from build123d import *

# Parameters (mm, degrees)
F0_W           = 51
F0_H           = 56
F0_W_2         = 47
F0_H_2         = 52
F1_DEPTH       = 1.5
F2_R           = 5
F3_DEPTH       = 3
F5_D           = 2
F5_CBORE_D     = 3.7
F5_CBORE_DEPTH = 1
F7_DEPTH       = 1.5


with BuildPart() as f1:
    # F0 (on Front) → F1 (new body)
    with BuildSketch(Plane.XZ):
        with Locations((25.5, 28)):
            Rectangle(F0_W, F0_H)
        with Locations((25.5, 28)):
            Rectangle(F0_W_2, F0_H_2, mode=Mode.SUBTRACT)
        with Locations((25.5, 28)):
            Rectangle(F0_W_2, F0_H_2)
    extrude(amount=F1_DEPTH)

    # F2
    f2_edges = [f1.edges().sort_by_distance(p)[0] for p in [
        (0, -0.75, 56),
        (51, -0.75, 56),
        (51, -0.75, 0),
        (0, -0.75, 0),
    ]]
    fillet(f2_edges, radius=F2_R)

    # F0 (on Front) → F3 (join)
    with BuildSketch(Plane.XZ):
        with Locations((25.5, 28)):
            Rectangle(F0_W_2, F0_H_2)
    extrude(amount=F3_DEPTH)

    # F5 (through all)
    with Locations(Plane(origin=(0, 0, 0), x_dir=(1, 0, 0), z_dir=(0, 1, 0))):
        with Locations((47.75, -52.75), (3.25, -52.75), (47.75, -3.25), (3.25, -3.25)):
            CounterBoreHole(F5_D / 2, F5_CBORE_D / 2, F5_CBORE_DEPTH)

    # F6 (on face) → F7 (cut)
    with BuildSketch(Plane.XZ.offset(3)):
        with BuildLine():
            Line((2, 54), (2, 50.2))
            ThreePointArc((2, 50.2), (4.6870057685, 51.3129942315), (5.8, 54))
            Line((5.8, 54), (2, 54))
        make_face()
        with BuildLine():
            ThreePointArc((45.2, 54), (46.3129942315, 51.3129942315), (49, 50.2))
            Line((49, 50.2), (49, 54))
            Line((49, 54), (45.2, 54))
        make_face()
        with BuildLine():
            Line((49, 2), (49, 5.8))
            ThreePointArc((49, 5.8), (46.3129942315, 4.6870057685), (45.2, 2))
            Line((45.2, 2), (49, 2))
        make_face()
        with BuildLine():
            ThreePointArc((5.8, 2), (4.6870057685, 4.6870057685), (2, 5.8))
            Line((2, 5.8), (2, 2))
            Line((2, 2), (5.8, 2))
        make_face()
    extrude(amount=-F7_DEPTH, mode=Mode.SUBTRACT)


solid = f1.part
Read the model definition and answer for the solid it produces. Units are mm, in the model's axes. A direction names the side the tool comes from. Round coordinates to 2 decimals unless told otherwise and drop trailing zeros. Write each loop counter-clockwise with the first axis right and the second up, starting at its lowest first coordinate (ties: lowest second). Pieces come first, ordered by that corner, then holes. Notation, with made-up numbers: (37, 23) - (85, 23) arc R35 ccw to (85, 62) - close; hole circle Ø2 at (33, 78.5). An arc over 180 degrees is marked (long way). One line per question, with ' | ' between items. Start each with the question number.
1. Section C-C (x = 3.25) is taken. Determine the outline of the cut face in (y, z).
2. For a pull along Z with two mould halves and no side action, classify faces 1 (the face through (1, -1, 54)), 2 (the face through (49, -1, 1)), 3 (the face through (47.21, -1.25, 51.91)), 4 (the face through (0, -1, 28)) as +Z half, -Z half, draft (parallel to the pull), parting line (faces both ways), or undercut.
3. For faces 5 (the face through (46.284, -2.26, 51.343)), 6 (the face through (46.343, -2.26, 4.716)), 7 (the face through (1, -1.5, 30)), 8 (the face through (2.849, -0.493, 54.556)), 9 (the face through (4.716, -2.26, 4.657)), determine the directions among +Z, -Z, +X, -X, +Y, -Y from which every point of the face is accessible in a straight line to the end or side of a thin tool.
4. Find the intervals of material crossed by probe 1 along X at (y, z) = (-0.65, 3.5); probe 2 along X at (y, z) = (-1.25, 52.75); probe 3 along Z at (x, y) = (31.5, -2.55), in increasing order. Write a range as [from, to].
5. Section D-D (z = 52.75) is taken. Determine the outline of the cut face in (x, y), and give its area (3 significant figures).
6. Section B-B (z = 8.5) is taken. Determine the outline of the cut face in (x, y), and give its area (3 significant figures).
7. Section A-A (x = 14.5) is taken. Determine the outline of the cut face in (y, z).
8. Each of these flat-tipped pins is pushed along its axis until it touches: pin 1 (0.8 mm diameter, centred on y = -2.5, z = 22, fed in from -X); pin 2 (3.5 mm diameter, centred on x = 3.25, z = 3.25, fed in from -Y); pin 3 (0.8 mm diameter, centred on y = -2.5, z = 35.5, fed in from +X). Where does it stop, or does it pass through?
Filled in:
1) outline: (-3, 5.59) - (-1.5, 5.59) - (-1.5, 4.25) - (-1, 4.25) - (-1, 5.1) - (0, 5.1) - (0, 50.9) - (-1, 50.9) - (-1, 51.75) - (-1.5, 51.75) - (-1.5, 50.41) - (-3, 50.41) - close; (-1.5, 0.32) - (0, 0.32) - (0, 1.4) - (-1, 1.4) - (-1, 2.25) - (-1.5, 2.25) - close; (-1.5, 53.75) - (-1, 53.75) - (-1, 54.6) - (0, 54.6) - (0, 55.68) - (-1.5, 55.68) - close
2) face 1: +Z half | face 2: -Z half | face 3: undercut | face 4: draft
3) face 5: +Z, +X, -Y | face 6: -Z, +X, -Y | face 7: -Y | face 8: +Y | face 9: -Z, -X, -Y
4) probe 1: [0.23, 1.42], [5.08, 45.92], [49.58, 50.77] | probe 2: [0.32, 2.25], [4.25, 46.75], [48.75, 50.68] | probe 3: [2, 54]
5) outline: (0.32, -1.5) - (2.25, -1.5) - (2.25, -1) - (1.4, -1) - (1.4, 0) - (0.32, 0) - close; (4.25, -1.5) - (5.59, -1.5) - (5.59, -3) - (45.41, -3) - (45.41, -1.5) - (46.75, -1.5) - (46.75, -1) - (45.9, -1) - (45.9, 0) - (5.1, 0) - (5.1, -1) - (4.25, -1) - close; (48.75, -1.5) - (50.68, -1.5) - (50.68, 0) - (49.6, 0) - (49.6, -1) - (48.75, -1) - close | area: 126 mm²
6) outline: (0, -1.5) - (2, -1.5) - (2, -3) - (49, -3) - (49, -1.5) - (51, -1.5) - (51, 0) - (0, 0) - close | area: 147 mm²
7) outline: (-3, 2) - (-1.5, 2) - (-1.5, 0) - (0, 0) - (0, 56) - (-1.5, 56) - (-1.5, 54) - (-3, 54) - close
8) pin 1: x = 2 | pin 2: y = -1.5 | pin 3: x = 49
